For this review, use the dimensioned drawing (mm, ordinates from the lowest corner) and the shaded views. Coordinates: 2 decimals unless noted, no trailing zeros. Write each loop counter-clockwise with the first axis right and the second up, starting at its lowest first coordinate (ties: lowest second). Pieces come first, ordered by that corner, then holes. Notation, with made-up numbers: (76.5, -18.5) - (106.5, -18.5) arc R25 cw to (106.5, -0.5) - close; hole circle Ø6 at (-19, -33). An arc over 180 degrees is marked (long way). Use one line per item in the form item = value. Start each with the question number.
1) For L1, parallel to Y at x = 3, z = 2.9 (1 decimal); L2, parallel to X at y = 3.75, z = 4.35; L3, parallel to X at y = 3.25, z = 0.7, list the stretches that pass through material, from the lowest coordinate up. Write a range as from..to.
2) Insertion check: P1, Ø12, axis at x = 11.5, y = 12.5, coming from the -Z side; P2, Ø2.5, axis at x = 3, y = 15.3, coming from the +Z side. Each pin has a flat end and moves straight along its axis. Give the tip position at first contact, or say it passes through.
3) We need section A-A (z = 0.95). Give the boundary of the cut face in (x, y) (1 decimal).
4) Mouldability with a two-part tool opening along X and no side actions: class the marked faces 1, 2 and 3 as pulls with the +X half, pulls with the -X half, needs draft (parallel to the pull), parting line crosses it, or undercut.
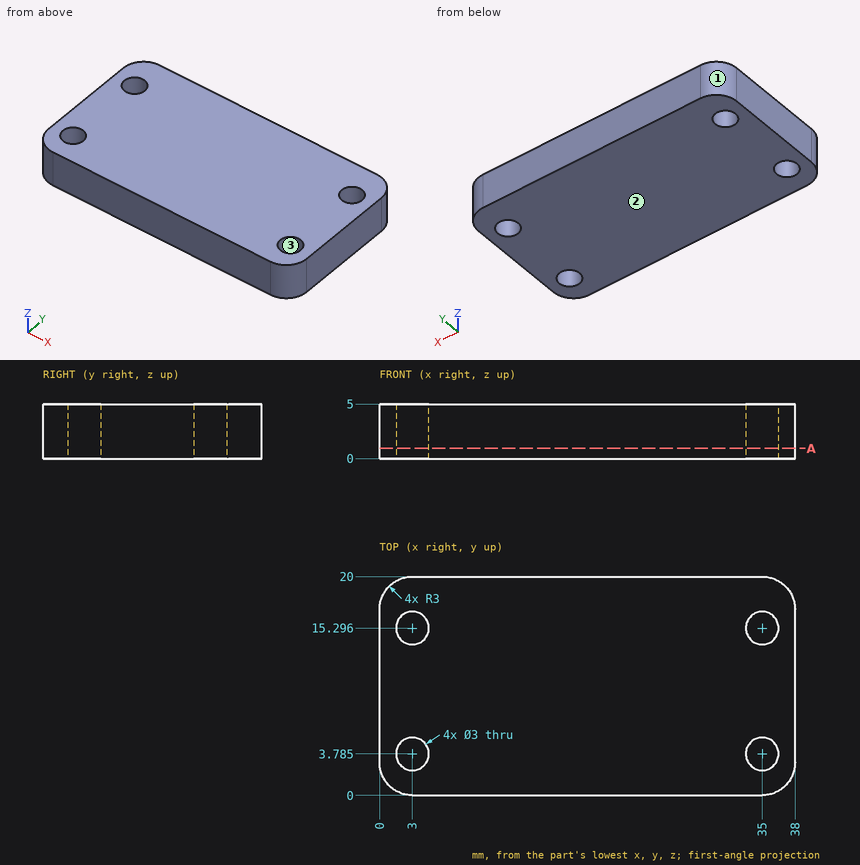
Determined:
q1.L1 = 0..2.3, 5.3..13.8, 16.8..20
q1.L2 = 0..1.5, 4.5..33.5, 36.5..38
q1.L3 = 0..1.6, 4.4..33.6, 36.4..38
q2.P1 = 0
q2.P2 = through
q3.outline = (0, 3) arc R3 ccw to (3, 0) - (35, 0) arc R3 ccw to (38, 3) - (38, 17) arc R3 ccw to (35, 20) - (3, 20) arc R3 ccw to (0, 17) - close; hole circle Ø3 at (3, 3.8); hole circle Ø3 at (3, 15.3); hole circle Ø3 at (35, 3.8); hole circle Ø3 at (35, 15.3)
q4.face_1 = pulls with the -X half
q4.face_2 = needs draft
q4.face_3 = undercut
